The drawing under review shows one solid part. Ordinate dimensions are in mm from its lowest x, y, z. Give positions to 0.01 mm unless a question says otherwise; leave off trailing zeros. Order: outer loops, then holes, each group sorted by start corner. A loop starts at its lowest first (then second) coordinate and runs counter-clockwise, first axis right, second up. Notation, with made-up numbers: (-7.75, -26.75) -> (29.25, -26.75) arc R9 ccw to (29.25, -20.75) -> close; hole circle Ø11 at (-12, -21.75). An arc over 180 degrees is marked (long way). One line per item, written item: value.
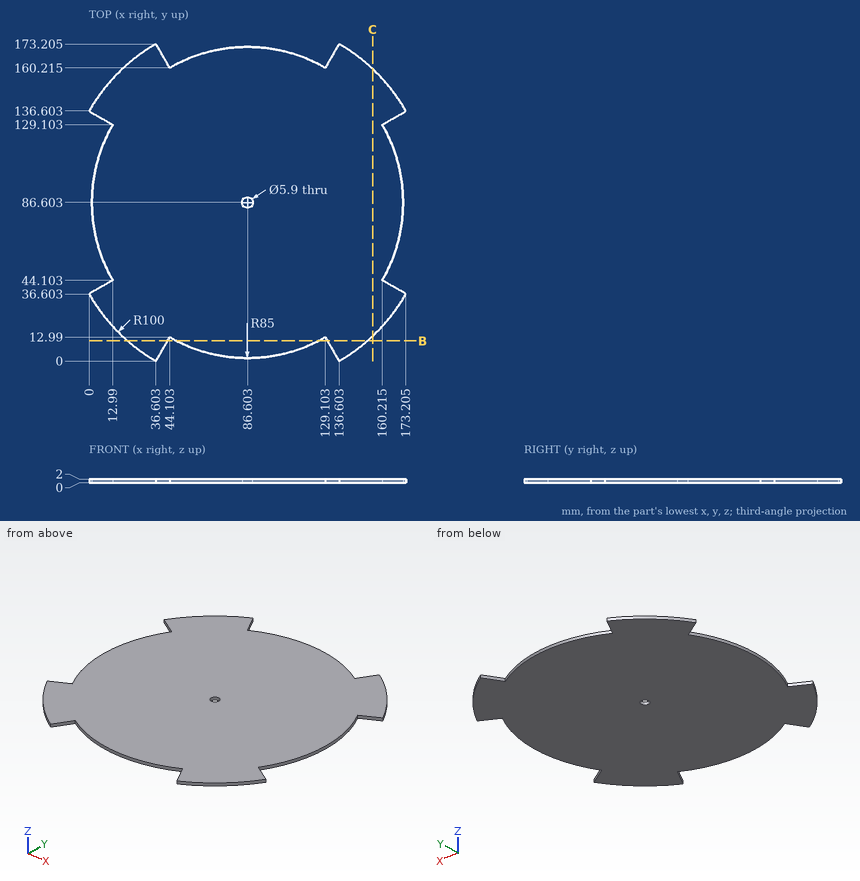
Item 1: To check wall thickness, follow line 1 along Y through (x, z) = (163.5, 0.9) (1 decimal); line 2 along Y through (x, z) = (84, 1.75) (1 decimal); line 3 along Y through (x, z) = (66.5, 0.35) (1 decimal). State the ranges of each line that lie inside material, in increasing order. Write a range as from..to.
Returned:
line 1: 22.7..42.2, 50.4..122.8, 131..150.5
line 2: 1.6..85.2, 88..171.6
line 3: 4..169.2
Item 2: Clearance check with a flat-ended pin moving along its axis: P1, Ø1, axis at x = 49, z = 0.5, coming from the +Y side. State where the tip first meets the part, or that it passes through.
Returned:
P1: y = 163.08
Item 3: Add section B-B on y = 11. Give the boundary of the cut face in (x, z).
Returned:
outline: (21.15, 0) -> (42.95, 0) -> (42.95, 2) -> (21.15, 2) -> close; (47.75, 0) -> (125.45, 0) -> (125.45, 2) -> (47.75, 2) -> close; (130.25, 0) -> (152.06, 0) -> (152.06, 2) -> (130.25, 2) -> close
Item 4: Add section C-C on x = 155. Give the boundary of the cut face in (y, z).
Returned:
outline: (13.65, 0) -> (159.55, 0) -> (159.55, 2) -> (13.65, 2) -> close
